Autodesk Inventor part; units mm, degrees
ref_plane "YZ Plane" through (0, 0, 0) normal (1, 0, 0) x (0, 1, 0)
ref_plane "XZ Plane" through (0, 0, 0) normal (0, 1, 0) x (-1, 0, 0)
ref_plane "XY Plane" through (0, 0, 0) normal (0, 0, 1) x (1, 0, 0)
sketch "Sketch1" plane through (0, 0, 0) normal (0, 1, 0) x (-1, 0, 0)
  line L0 (0, 0) -> (30, 0)
  line L1 (30, 0) -> (30, -3)
  line L2 (30, -3) -> (0, -3)
  line L3 (0, -3) -> (0, 0)
  dimension "d0" = 30
  dimension "d1" = 3
extrude "Extrusion1" add sketch "Sketch1" along normal blind 7.5
sketch "Sketch2" plane through (0, 7.5, 0) normal (0, 1, 0) x (1, 0, 0)
  circle A0 centre (-2.5481, 1.391) radius 1.0387
  point P0 (0, 0)
extrude "Extrusion2" cut sketch "Sketch2" against normal blind 0.1
sketch "Sketch3" plane through (-30, 0, 0) normal (0, 0, 1) x (1, 0, 0)
  circle A0 centre (26.5, 2.5) radius 0.6105
  line L0 (0, 0) -> (30, 0)
  line L1 (30, 0) -> (30, 7.5)
  circle A1 centre (22, 2.5) radius 1.95
  circle A2 centre (17.5, 2.5) radius 0.6105
  line L2 (30, 7.5) -> (0, 7.5)
  line L3 (0, 7.5) -> (30, 7.5)
  line L4 (30, 7.5) -> (15, 7.5)
  line L5 (15, 7.5) -> (15, 0)
  circle A3 centre (3.5, 2.5) radius 0.6105
  circle A4 centre (8, 2.5) radius 1.95
  circle A5 centre (12.5, 2.5) radius 0.6105
  dimension "d6" = 1.221
  dimension "d7" = 2.5
  dimension "d8" = 3.5
  dimension "d9" = 3.9
  dimension "d10" = 8
  dimension "d11" = 1.221
  dimension "d12" = 2.5
  dimension "d13" = 4.5
extrude "Extrusion3" cut sketch "Sketch3" against normal blind 3 contours A0 | A1 | A2 | A3 | A4 | A5
properties part number "backmidmotorwall"
Read the model definition and answer for the solid it produces. Units are mm, in the model's axes. A direction names the side the tool comes from. Give positions to 0.01 mm unless a question says otherwise; leave off trailing zeros. Loops run counter-clockwise (first coordinate to the right, second up) from the corner with the lowest first, then second, coordinate; pieces in that order, holes last. Notation, with made-up numbers: (70, 63) -> (102, 63) arc R31 cw to (102, 96) -> close; hole circle Ø4 at (71.25, -30.75). An arc over 180 degrees is marked (long way). Use a Markdown table: item, result.
Q1. A tool of negligible diameter and unlimited length cuts with its end or side. For faces 4 (the face through (-3, 7.4, -1)), 5 (the face through (-15, 4, 0)), from which of +Z, -Z, +X, -X, +Y, -Y can it reach the whole face along a straight path? Write none if from no direction.
Solved:
| item | result |
|---|---|
| face 4 | +Y |
| face 5 | +Z, +X, -X, +Y, -Y |
Q2. Determine the mould class of faces 1 (the face through (-12.172, 3.015, -1.479)), 2 (the face through (0, 4, -2)), 3 (the face through (-15, 0, -1)) for opening direction X: pulls with the +X half, pulls with the -X half, needs draft (parallel to the pull), parting line crosses it, or undercut.
Solved:
| item | result |
|---|---|
| face 1 | undercut |
| face 2 | pulls with the +X half |
| face 3 | needs draft |
Q3. Section A-A, the plane x = -26.5 is taken. Determine the outline of the cut face in (y, z).
Solved:
| item | result |
|---|---|
| outline | (0, -3) -> (1.89, -3) -> (1.89, 0) -> (0, 0) -> close; (3.11, -3) -> (7.5, -3) -> (7.5, 0) -> (3.11, 0) -> close |
Q4. Section C-C, the plane x = -8 is taken. Determine the outline of the cut face in (y, z), then the cut area to 3 significant figures.
Solved:
| item | result |
|---|---|
| outline | (0, -3) -> (0.55, -3) -> (0.55, 0) -> (0, 0) -> close; (4.45, -3) -> (7.5, -3) -> (7.5, 0) -> (4.45, 0) -> close |
| area | 10.8 mm^2 |
Q5. Find the intervals of material crossed by line 1 along Y through (x, z) = (-22, -1.65); line 2 along X through (y, z) = (4, -2.25); line 3 along X through (y, z) = (1.5, -2.7), in increasing order.
Solved:
| item | result |
|---|---|
| line 1 | y = 0 to 0.55, 4.45 to 7.5 |
| line 2 | x = -30 to -23.25, -20.75 to -9.25, -6.75 to 0 |
| line 3 | x = -30 to -23.67, -20.33 to -9.67, -6.33 to 0 |
Q6. Each of these flat-tipped pins is pushed along its axis until it touches: pin 1 (2 mm diameter, centred on x = -17.5, y = 2.5, fed in from +Z); pin 2 (0.6 mm diameter, centred on x = -2.5, z = -1.5, fed in from +Y). Where does it stop, or does it pass through?
Solved:
| item | result |
|---|---|
| pin 1 | stops at z = 0 |
| pin 2 | stops at y = 7.4 |
Q7. Section D-D, the plane z = -1 is taken. Determine the outline of the cut face in (x, y).
Solved:
| item | result |
|---|---|
| outline | (-30, 0) -> (0, 0) -> (0, 7.5) -> (-1.59, 7.5) -> (-1.59, 7.4) -> (-3.51, 7.4) -> (-3.51, 7.5) -> (-30, 7.5) -> close; hole circle Ø1.22 at (-26.5, 2.5); hole circle Ø3.9 at (-22, 2.5); hole circle Ø1.22 at (-17.5, 2.5); hole circle Ø1.22 at (-12.5, 2.5); hole circle Ø3.9 at (-8, 2.5); hole circle Ø1.22 at (-3.5, 2.5) |
Q8. Section B-B, the plane z = -2.7 is taken. Determine the outline of the cut face in (x, y), then the cut area to 3 significant figures.
Solved:
| item | result |
|---|---|
| outline | (-30, 0) -> (0, 0) -> (0, 7.5) -> (-30, 7.5) -> close; hole circle Ø1.22 at (-26.5, 2.5); hole circle Ø3.9 at (-22, 2.5); hole circle Ø1.22 at (-17.5, 2.5); hole circle Ø1.22 at (-12.5, 2.5); hole circle Ø3.9 at (-8, 2.5); hole circle Ø1.22 at (-3.5, 2.5) |
| area | 196 mm^2 |
